from build123d import *

# Parameters (mm, degrees)
F0_R     = 5
F1_DEPTH = 40


with BuildPart() as f1:
    # F0 (on Front) → F1 (new body)
    with BuildSketch(Plane.XZ):
        Polygon((-20, 23.076462), (-63.196195, 107.349918), (-119.260357, 78.613011), (-35.396944, -85), (-12.331214, -40), (-20, -40), align=None)
        Polygon((-12.331214, -40), (-35.396944, -85), (0, -154.057537), (35.396944, -85), (12.331214, -40), align=None)
        with Locations((0, -85)):
            Circle(F0_R, mode=Mode.SUBTRACT)
        Polygon((0, -154.057537), (-35.396944, -85), (-325, -650), (-254.206111, -650), align=None)
        Polygon((35.396944, -85), (0, -154.057537), (254.206111, -650), (325, -650), align=None)
        Polygon((20, -40), (12.331214, -40), (35.396944, -85), (114.1444, 68.632054), (58.080238, 97.368961), (20, 23.076462), align=None)
    extrude(amount=F1_DEPTH)


solid = f1.part
Verification items for the finished model (mm, model axes). A direction names the side the tool comes from. Coordinates: 2 decimals unless noted, no trailing zeros. Order: outer loops, then holes, each group sorted by start corner. A loop starts at its lowest first (then second) coordinate and runs counter-clockwise, first axis right, second up. Notation, with made-up numbers: M 24,-6.75 L 57,-6.75 A28 ccw 57,32.25 Z; hole C 38.25,32 d11. An arc over 180 degrees is marked long. Return JSON: item names as keys, results as strings.
1) Thickness scan on L1, parallel to Z at x = 0, y = -14.5; L2, parallel to X at y = -36, z = -569; L3, parallel to X at y = -25, z = -244. Record the ranges inside material, lowest first. Write a range as [from, to].
Answer list:
{"L1": "[-154.06, -90], [-80, -40]", "L2": "[-283.48, -212.69], [212.69, 283.48]", "L3": "[-116.9, -46.1], [46.1, 116.9]"}
2) Cross-section at D-D, the plane x = -165. Record the boundary of the cut face in (y, z).
Answer list:
{"outline": "M -40,-475.96 L 0,-475.96 L 0,-337.85 L -40,-337.85 Z"}
3) Cross-section at B-B, the plane z = -2. Record the boundary of the cut face in (x, y).
Answer list:
{"outline": "M -77.94,-40 L -20,-40 L -20,0 L -77.94,0 Z; M 20,-40 L 77.94,-40 L 77.94,0 L 20,0 Z"}
4) Cross-section at C-C, the plane z = -486. Record the boundary of the cut face in (x, y).
Answer list:
{"outline": "M -240.94,-40 L -170.14,-40 L -170.14,0 L -240.94,0 Z; M 170.14,-40 L 240.94,-40 L 240.94,0 L 170.14,0 Z"}
5) Release check for a two-part mould opening along X. For faces 6 (the flat face through (-77.916, -19.72, -2.048)), 7 (the flat face through (-50, -40, -242)), 8 (the flat face through (-128.882, -19.72, -405.5)) record: +X half, -X half, draft (parallel to the pull), parting line (faces both ways), or undercut.
Answer list:
{"face 6": "-X half", "face 7": "draft", "face 8": "undercut"}
6) Cross-section at A-A, the plane y = -22.5. Record the boundary of the cut face in (x, z), and give its area (3 significant figures).
Answer list:
{"outline": "M -325,-650 L -254.21,-650 L 0,-154.06 L 254.21,-650 L 325,-650 L 35.4,-85 L 114.14,68.63 L 58.08,97.37 L 20,23.08 L 20,-40 L -20,-40 L -20,23.08 L -63.2,107.35 L -119.26,78.61 L -35.4,-85 Z; hole C 0,-85 d10", "area": "97,800 mm2"}
7) Gauge pin test, flat ends, axial feed: pin 1 (5 mm diameter, centred on y = -35, z = -544, fed in from -X); pin 2 (12 mm diameter, centred on x = 188.5, y = -10, fed in from +Z); pin 3 (6 mm diameter, centred on y = -27, z = -508.5, fed in from +X). Record the tip position at first contact, or that the pin passes through.
Answer list:
{"pin 1": "x = -271.95", "pin 2": "z = -371.99", "pin 3": "x = 254.01"}
8) Access from +Z, -Z, +X, -X, +Y, -Y to the whole of each face (thin tool, end or side, straight path). Record for faces 1 (the flat face through (-178.171, -19.72, -363.545)), 2 (the flat face through (125.324, -19.72, -398.557)), 3 (the flat face through (182.226, -19.72, -371.455)), 4 (the flat face through (-290, -20, -650)), 5 (the flat face through (0, -20, -40)).
Answer list:
{"face 1": "-X, +Y, -Y", "face 2": "-Z, +Y, -Y", "face 3": "+X, +Y, -Y", "face 4": "-Z, +X, -X, +Y, -Y", "face 5": "+Z, +Y, -Y"}
